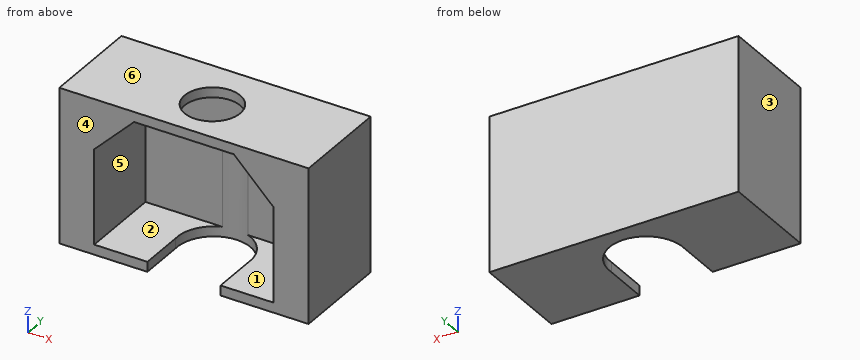
```python
from build123d import *

# Parameters (mm, degrees)
F0_W     = 30
F0_H     = 18.6
F1_DEPTH = 12
F3_START = 7.4
F2_R     = 3.35
F3_DEPTH = 27.8
F4_DEPTH = 2.1
F5_DEPTH = 11.2


with BuildPart() as f1:
    # F0 (on Front) → F1 (new body)
    with BuildSketch(Plane.XZ):
        with Locations((-15, 9.3)):
            Rectangle(F0_W, F0_H)
        Polygon((-21, 17.4), (-15, 17.4), (-9, 17.4), (-4.2, 17.4), (-4.2, 12.6), (-4.2, 9.3), (-4.2, 1.2), (-15, 1.2), (-25.8, 1.2), (-25.8, 9.3), (-25.8, 12.6), (-25.8, 17.4), align=None, mode=Mode.SUBTRACT)
        Polygon((-25.8, 12.6), (-21, 17.4), (-25.8, 17.4), align=None)
        Polygon((-4.2, 17.4), (-9, 17.4), (-4.2, 12.6), align=None)
    extrude(amount=F1_DEPTH)

    # F2 (on Top) → F3 (cut)
    with BuildSketch(Plane.XY.offset(F3_START)):
        with Locations((-15, -6.5)):
            Circle(F2_R)
    extrude(amount=F3_DEPTH, mode=Mode.SUBTRACT)

    # F0 (on Front) → F4 (join)
    with BuildSketch(Plane.XZ):
        Polygon((-9, 17.4), (-15, 17.4), (-21, 17.4), (-25.8, 12.6), (-25.8, 9.3), (-25.8, 1.2), (-15, 1.2), (-4.2, 1.2), (-4.2, 9.3), (-4.2, 12.6), align=None)
    extrude(amount=F4_DEPTH)

    # F2 (on Top) → F5 (cut)
    with BuildSketch(Plane.XY):
        with BuildLine():
            Line((-19.3997538172, -14.9291978362), (-18.3492293667, -15.2891640001))
            Line((-18.3492293667, -15.2891640001), (-15, -14.3958181143))
            Line((-15, -14.3958181143), (-11.6507706333, -15.2891640001))
            Line((-11.6507706333, -15.2891640001), (-10.6002461828, -14.9291978362))
            Line((-10.6002461828, -14.9291978362), (-10.6002461828, -6.5465440438))
            ThreePointArc((-10.6002461828, -6.5465440438), (-15, -10.9), (-19.3997538172, -6.5465440438))
            Line((-19.3997538172, -6.5465440438), (-19.3997538172, -14.9291978362))
        make_face()
        with BuildLine():
            ThreePointArc((-10.6002461828, -6.5465440438), (-15, -1.8248851289), (-19.3997538172, -6.5465440438))
            ThreePointArc((-19.3997538172, -6.5465440438), (-15.0232723474, -2.1000615461), (-10.6, -6.5))
            ThreePointArc((-10.6, -6.5), (-10.6000615461, -6.5232723474), (-10.6002461828, -6.5465440438))
        make_face()
        with BuildLine():
            ThreePointArc((-10.6, -6.5), (-15.0232723474, -2.1000615461), (-19.3997538172, -6.5465440438))
            ThreePointArc((-19.3997538172, -6.5465440438), (-15, -10.9), (-10.6002461828, -6.5465440438))
            ThreePointArc((-10.6002461828, -6.5465440438), (-10.6000615461, -6.5232723474), (-10.6, -6.5))
        make_face()
        with Locations((-15, -6.5)):
            Circle(F2_R, mode=Mode.SUBTRACT)
        with Locations((-15, -6.5)):
            Circle(F2_R)
    extrude(amount=F5_DEPTH, mode=Mode.SUBTRACT)


solid = f1.part
```
Build history of the part. All positions in model axes, mm. Face numbers are marked on the shaded views. A direction names the side the tool comes from. Give positions to 0.01 mm unless a question says otherwise; leave off trailing zeros. Loops run counter-clockwise (first coordinate to the right, second up) from the corner with the lowest first, then second, coordinate; pieces in that order, holes last. Notation, with made-up numbers: (86.25, -1) - (98.25, -1) arc R18 ccw to (98.25, 4) - close; hole circle Ø4 at (71.5, -10). An arc over 180 degrees is marked (long way). Use a Markdown table: item, result.
(1) Which spindle directions (+Z, -Z, +X, -X, +Y, -Y) get a long thin tool onto all of the face, cutting with end or side? Do the marked faces 5 and 6. Say none if no direction does.
Taken from the geometry:
| item | result |
|---|---|
| face 5 | -Y |
| face 6 | +Z, +X, -X, +Y, -Y |
(2) Drop flat-ended pins along their axis: pin 1 Ø2 at (x, y) = (-12.5, -10.5) entering from -Z; pin 2 Ø5 at (x, z) = (-11.5, 10.5) entering from -Y. Give the stop position or say it passes through.
Taken from the geometry:
| item | result |
|---|---|
| pin 1 | z = 17.4 |
| pin 2 | y = -2.1 |
(3) Band-saw the part on B-B (z = 8.75). Give the cut face in (x, y).
Taken from the geometry:
| item | result |
|---|---|
| outline | (-30, -12) - (-25.8, -12) - (-25.8, -2.1) - (-16.53, -2.1) arc R4.41 cw to (-13.47, -2.1) - (-4.2, -2.1) - (-4.2, -12) - (0, -12) - (0, 0) - (-30, 0) - close |
(4) Band-saw the part on D-D (x = -7.5). Give the cut face in (y, z).
Taken from the geometry:
| item | result |
|---|---|
| outline | (-12, 0) - (0, 0) - (0, 18.6) - (-12, 18.6) - (-12, 15.9) - (-2.1, 15.9) - (-2.1, 1.2) - (-12, 1.2) - close |
(5) Band-saw the part on C-C (y = -4.5). Give the cut face in (x, z), and give its area (3 significant figures).
Taken from the geometry:
| item | result |
|---|---|
| outline | (-30, 0) - (-19.05, 0) - (-19.05, 1.2) - (-25.8, 1.2) - (-25.8, 12.6) - (-21, 17.4) - (-17.69, 17.4) - (-17.69, 18.6) - (-30, 18.6) - close; (-12.31, 17.4) - (-9, 17.4) - (-4.2, 12.6) - (-4.2, 1.2) - (-10.95, 1.2) - (-10.95, 0) - (0, 0) - (0, 18.6) - (-12.31, 18.6) - close |
| area | 215 mm2 |
(6) Wall check: line 1 along X through (y, z) = (-6.5, 18.1); line 2 along Y through (x, z) = (-15, 18.3); line 3 along Z through (x, y) = (-20, -6). Give the ranges that are in metal, low to high.
Taken from the geometry:
| item | result |
|---|---|
| line 1 | -30 to -18.35, -11.65 to 0 |
| line 2 | -12 to -9.85, -3.15 to 0 |
| line 3 | 0 to 1.2, 17.4 to 18.6 |
(7) Pull direction X, two halves, no side cores. Call the marked faces 1, 2, 3 and 4: +X half, -X half, draft (parallel to the pull), parting line (faces both ways), or undercut.
Taken from the geometry:
| item | result |
|---|---|
| face 1 | undercut |
| face 2 | undercut |
| face 3 | -X half |
| face 4 | draft |
(8) Band-saw the part on A-A (x = -15). Give the cut face in (y, z), and give its area (3 significant figures).
Taken from the geometry:
| item | result |
|---|---|
| outline | (-12, 17.4) - (-9.85, 17.4) - (-9.85, 18.6) - (-12, 18.6) - close; (-3.15, 17.4) - (-2.1, 17.4) - (-2.1, 11.2) - (-1.82, 11.2) - (-1.82, 0) - (0, 0) - (0, 18.6) - (-3.15, 18.6) - close |
| area | 39.8 mm2 |
